```python
from build123d import *

# Parameters (mm, degrees)
F1_DEPTH    = 5
F2_T1_DEPTH = 5
F2_T3_DEPTH = 5
F3_T1_DEPTH = 6.2324692544
F3_T3_DEPTH = 6.2324692544
F4_R        = 1.65
F5_DEPTH    = 11.501
F6_SIZE     = 0.5


# Not quite as in the source:
# - a fillet or chamfer that OpenCascade refuses, or shapes differently, is made with other operations: its cross-section is extruded or revolved along the edge and cut away or added
# - a pattern or mirror of a feature is missing from the dataset's text; its kind, count and spacing are read off the source's solid


with BuildPart() as f1:
    # F0 (on Front) → F1 (new body, symmetric)
    with BuildSketch(Plane.XZ):
        with BuildLine():
            Line((4.8989794856, 1), (23.5, 1))
            Line((23.5, 1), (23.5, 12.5))
            Line((23.5, 12.5), (16.5, 12.5))
            Line((16.5, 12.5), (16.5, 4))
            Line((16.5, 4), (6.9282032303, 4))
            ThreePointArc((6.9282032303, 4), (4, 6.9282032303), (0, 8))
            ThreePointArc((0, 8), (-4, 6.9282032303), (-6.9282032303, 4))
            Line((-6.9282032303, 4), (-16.5, 4))
            Line((-16.5, 4), (-16.5, 12.5))
            Line((-16.5, 12.5), (-23.5, 12.5))
            Line((-23.5, 12.5), (-23.5, 1))
            Line((-23.5, 1), (-4.8989794856, 1))
            ThreePointArc((-4.8989794856, 1), (-3.1622776602, 3.8729833462), (0, 5))
            ThreePointArc((0, 5), (3.1622776602, 3.8729833462), (4.8989794856, 1))
        make_face()
    extrude(amount=F1_DEPTH, both=True)

    # F2: fillet of radius 7 on 8 edges, made by hand

    # F2_s2 → F2_t1 (join)
    with BuildSketch(Plane.XZ.offset(-5)):
        with BuildLine():
            ThreePointArc((16.5, 11), (14.4497474683, 6.0502525317), (9.5, 4))
            Line((9.5, 4), (16.5, 4))
            Line((16.5, 4), (16.5, 11))
        make_face()
        with BuildLine():
            ThreePointArc((10.1980390272, 4), (7.6420004255, 4.4833546462), (5.4389541478, 5.8666666667))
            ThreePointArc((5.4389541478, 5.8666666667), (6.2536194731, 4.989212712), (6.9282032303, 4))
            Line((6.9282032303, 4), (10.1980390272, 4))
        make_face()
        with BuildLine():
            ThreePointArc((-5.4389541478, 5.8666666667), (-7.6420004255, 4.4833546462), (-10.1980390272, 4))
            Line((-10.1980390272, 4), (-6.9282032303, 4))
            ThreePointArc((-6.9282032303, 4), (-6.2536194731, 4.989212712), (-5.4389541478, 5.8666666667))
        make_face()
        with BuildLine():
            ThreePointArc((-9.5, 4), (-14.4497474683, 6.0502525317), (-16.5, 11))
            Line((-16.5, 11), (-16.5, 4))
            Line((-16.5, 4), (-9.5, 4))
        make_face()
    extrude(amount=F2_T1_DEPTH)

    # F2_s4 → F2_t3 (join)
    with BuildSketch(Plane.XZ):
        with BuildLine():
            ThreePointArc((16.5, 11), (14.4497474683, 6.0502525317), (9.5, 4))
            Line((9.5, 4), (16.5, 4))
            Line((16.5, 4), (16.5, 11))
        make_face()
        with BuildLine():
            ThreePointArc((10.1980390272, 4), (7.6420004255, 4.4833546462), (5.4389541478, 5.8666666667))
            ThreePointArc((5.4389541478, 5.8666666667), (6.2536194731, 4.989212712), (6.9282032303, 4))
            Line((6.9282032303, 4), (10.1980390272, 4))
        make_face()
        with BuildLine():
            ThreePointArc((-5.4389541478, 5.8666666667), (-7.6420004255, 4.4833546462), (-10.1980390272, 4))
            Line((-10.1980390272, 4), (-6.9282032303, 4))
            ThreePointArc((-6.9282032303, 4), (-6.2536194731, 4.989212712), (-5.4389541478, 5.8666666667))
        make_face()
        with BuildLine():
            ThreePointArc((-9.5, 4), (-14.4497474683, 6.0502525317), (-16.5, 11))
            Line((-16.5, 11), (-16.5, 4))
            Line((-16.5, 4), (-9.5, 4))
        make_face()
    extrude(amount=F2_T3_DEPTH)

    # F3: chamfer of 0.5 on 4 edges, made by hand

    # F3_s2 → F3_t1 (cut)
    with BuildSketch(Plane.XZ.offset(-6.2324692544)):
        with BuildLine():
            Line((-4.7731743681, 1.4483837223), (-5.3918225964, 0.9880608955))
            Line((-5.3918225964, 0.9880608955), (-5.3918225964, 0.9780608955))
            ThreePointArc((-5.3918225964, 0.9780608955), (-5.145401041, 0.99), (-4.8989794856, 0.99))
            Line((-4.8989794856, 0.99), (-4.8891815266, 0.998))
            ThreePointArc((-4.8891815266, 0.998), (-4.8374189809, 1.2245315852), (-4.7635959284, 1.445510833))
            Line((-4.7635959284, 1.445510833), (-4.7731743681, 1.4483837223))
        make_face()
        with BuildLine():
            Line((4.7731743681, 1.4483837223), (5.3918225964, 0.9880608955))
            Line((5.3918225964, 0.9880608955), (5.3918225964, 0.9780608955))
            ThreePointArc((5.3918225964, 0.9780608955), (5.145401041, 0.99), (4.8989794856, 0.99))
            Line((4.8989794856, 0.99), (4.8891815266, 0.998))
            ThreePointArc((4.8891815266, 0.998), (4.8374189809, 1.2245315852), (4.7635959284, 1.445510833))
            Line((4.7635959284, 1.445510833), (4.7731743681, 1.4483837223))
        make_face()
    extrude(amount=F3_T1_DEPTH, mode=Mode.SUBTRACT)

    # F3_s4 → F3_t3 (cut)
    with BuildSketch(Plane.XZ):
        with BuildLine():
            Line((-4.7731743681, 1.4483837223), (-5.3918225964, 0.9880608955))
            Line((-5.3918225964, 0.9880608955), (-5.3918225964, 0.9780608955))
            ThreePointArc((-5.3918225964, 0.9780608955), (-5.145401041, 0.99), (-4.8989794856, 0.99))
            Line((-4.8989794856, 0.99), (-4.8891815266, 0.998))
            ThreePointArc((-4.8891815266, 0.998), (-4.8374189809, 1.2245315852), (-4.7635959284, 1.445510833))
            Line((-4.7635959284, 1.445510833), (-4.7731743681, 1.4483837223))
        make_face()
        with BuildLine():
            Line((4.7731743681, 1.4483837223), (5.3918225964, 0.9880608955))
            Line((5.3918225964, 0.9880608955), (5.3918225964, 0.9780608955))
            ThreePointArc((5.3918225964, 0.9780608955), (5.145401041, 0.99), (4.8989794856, 0.99))
            Line((4.8989794856, 0.99), (4.8891815266, 0.998))
            ThreePointArc((4.8891815266, 0.998), (4.8374189809, 1.2245315852), (4.7635959284, 1.445510833))
            Line((4.7635959284, 1.445510833), (4.7731743681, 1.4483837223))
        make_face()
    extrude(amount=F3_T3_DEPTH, mode=Mode.SUBTRACT)

    # F4 (on face) → F5 (cut, through all)
    with BuildSketch(Plane.XY.offset(12.5)):
        with Locations((19.5, 0)):
            Circle(F4_R)
    f5 = extrude(amount=-F5_DEPTH, mode=Mode.SUBTRACT)

    # F5_copies: F5 across plane
    add(f5.mirror(Plane(origin=(0, 0, 0), x_dir=(0, 0, -1), z_dir=(-1, 0, 0))), mode=Mode.SUBTRACT)

    # F6
    f6_edges = [f1.edges().sort_by_distance(p)[0] for p in [
        (19.5, 1.65, 12.5),
        (19.5, -1.65, 12.5),
        (19.5, 1.65, 1),
        (-19.5, 1.65, 1),
        (-19.5, 1.65, 12.5),
        (19.5, -1.65, 1),
        (-19.5, -1.65, 1),
        (-19.5, -1.65, 12.5),
    ]]
    chamfer(f6_edges, length=F6_SIZE)


solid = f1.part
```
Verification items for the finished model (mm, model axes). A direction names the side the tool comes from. Round coordinates to 2 decimals unless told otherwise and drop trailing zeros. Order: outer loops, then holes, each group sorted by start corner. A loop starts at its lowest first (then second) coordinate and runs counter-clockwise, first axis right, second up.
1) Tool access check on faces 4 (the flat face through (-23.5, 0, 7)), 5 (the cylindrical face through (14.623, 0.07, 6.229)). Record the directions out of +Z, -Z, +X, -X, +Y, -Y that give a thin tool (end or side, any length) a straight path to the whole face; none if there is none.
Geometry says:
face 4: +Z, -Z, -X, +Y, -Y
face 5: +Z, +Y, -Y
2) Depth check by flat-ended pin: pin 1 (3 mm diameter, centred on x = -19.5, y = 0, fed in from -Z); pin 2 (1 mm diameter, centred on x = 9.5, y = 1.5, fed in from +Z); pin 3 (1.5 mm diameter, centred on x = -2.5, y = 0, fed in from +Z). Enter the tip coordinate at first touch or a pass-through.
Geometry says:
pin 1: passes through
pin 2: stops at z = 4.1
pin 3: stops at z = 7.81
3) Material ranges on line 1 (Y direction, x = -19.5, z = 6.75); line 2 (X direction, y = -1, z = 3.25); line 3 (X direction, y = -0.25, z = 3.25), recorded low to high.
Geometry says:
line 1: y = -5 to -1.65, 1.65 to 5
line 2: x = -23.5 to -20.81, -18.19 to -3.8, 3.8 to 18.19, 20.81 to 23.5
line 3: x = -23.5 to -21.13, -17.87 to -3.8, 3.8 to 17.87, 21.13 to 23.5
4) Cross-section at B-B, the plane x = -19.5. Record the cut outline in (y, z), plus the area to 4 significant figures.
Geometry says:
outline: (-5, 1) - (-2.15, 1) - (-1.65, 1.5) - (-1.65, 12) - (-2.15, 12.5) - (-5, 12.5) - close; (1.65, 1.5) - (2.15, 1) - (5, 1) - (5, 12.5) - (2.15, 12.5) - (1.65, 12) - close
area: 76.55 mm2
5) Draft check along Y on faces 1 (the flat face through (0, 5, 6)), 2 (the cylindrical face through (-18.19, -1, 6.82)), 3 (the flat face through (23.5, 0, 7)). Enter one of: +Y half, -Y half, draft (parallel to the pull), parting line (faces both ways), or undercut.
Geometry says:
face 1: +Y half
face 2: undercut
face 3: draft
6) Cross-section at D-D, the plane z = 6.5. Record the cut outline in (x, y), plus the area to 3 significant figures.
Geometry says:
outline: (-23.5, -5) - (-14.86, -5) - (-14.86, 5) - (-23.5, 5) - close; (-4.66, -5) - (4.66, -5) - (4.66, 5) - (-4.66, 5) - close; (14.86, -5) - (23.5, -5) - (23.5, 5) - (14.86, 5) - close; hole circle Ø3.3 at (-19.5, 0); hole circle Ø3.3 at (19.5, 0)
area: 249 mm2
7) Cross-section at C-C, the plane y = 0. Give the number of separate pieces and of enclosed holes in the cut face, plus the area to 3 significant figures.
Geometry says:
separate pieces: 3
enclosed holes: 0
area: 216 mm2
8) Cross-section at A-A, the plane z = 2.5. Record the cut outline in (x, y), plus the area to 3 significant figures.
Geometry says:
outline: (-23.5, -5) - (-4.33, -5) - (-4.33, 5) - (-23.5, 5) - close; (4.33, -5) - (23.5, -5) - (23.5, 5) - (4.33, 5) - close; hole circle Ø3.3 at (-19.5, 0); hole circle Ø3.3 at (19.5, 0)
area: 366 mm2
